from build123d import *

# Parameters (mm, degrees)
SKETCH1_W                = 4.5
SKETCH1_H                = 3.5
BOSS_EXTRUDE1_DEPTH      = 4.5
SKETCH2_W                = 4
SKETCH2_H                = 3
CUT_EXTRUDE1_DEPTH       = 4.25
SKETCH3_R                = 0.15
BOSS_EXTRUDE2_DEPTH      = 2.7
BOSS_EXTRUDE2_DEPTH_BACK = 4
SKETCH4_W                = 3.5
SKETCH4_H                = 0.4
CUT_EXTRUDE2_DEPTH       = 5.5


with BuildPart() as part:
    # Sketch1 → Boss-Extrude1 (new body)
    with BuildSketch(Plane.XY):
        Rectangle(SKETCH1_W, SKETCH1_H)
    extrude(amount=BOSS_EXTRUDE1_DEPTH)

    # Sketch2 → Cut-Extrude1 (cut)
    with BuildSketch(Plane.XY.offset(4.5)):
        Rectangle(SKETCH2_W, SKETCH2_H)
    extrude(amount=-CUT_EXTRUDE1_DEPTH, mode=Mode.SUBTRACT)

    # Sketch3 → Boss-Extrude2 (add, two sides)
    with BuildSketch(Plane(origin=(0, 0, 0), x_dir=(-1, 0, 0), z_dir=(0, 0, -1))) as boss_extrude2_sk:
        with Locations((-0.75, -0.45)):
            Circle(SKETCH3_R)
        with Locations((0.75, -0.45)):
            Circle(SKETCH3_R)
    extrude(amount=BOSS_EXTRUDE2_DEPTH)
    extrude(boss_extrude2_sk.sketch, amount=-BOSS_EXTRUDE2_DEPTH_BACK)

    # Sketch4 → Cut-Extrude2 (cut, through all)
    with BuildSketch(Plane.ZY.offset(2.25)):
        with Locations((4.5, -0.45)):
            Rectangle(SKETCH4_W, SKETCH4_H)
    extrude(amount=-CUT_EXTRUDE2_DEPTH, mode=Mode.SUBTRACT)


solid = part.part
CAD build for the part. Positions are in the model's coordinates, mm. A direction names the side the tool comes from. Coordinates: 2 decimals unless noted, no trailing zeros. Order: outer loops, then holes, each group sorted by start corner. A loop starts at its lowest first (then second) coordinate and runs counter-clockwise, first axis right, second up.
Item 1: Two-plate mould, pull along X, no slides. Class faces 1 (the face through (0, 1.75, 2)), 2 (the face through (0, 1.5, 2)), 3 (the face through (-2, 0, 2)), 4 (the face through (2.25, 0, 2)): +X half, -X half, draft (parallel to the pull), parting line (faces both ways), or undercut.
Check sheet entries:
face 1: draft
face 2: undercut
face 3: undercut
face 4: +X half
Item 2: Drill centre lines: L1, parallel to X at y = 0.95, z = 2.75; L2, parallel to Y at x = -1.85, z = 2.5; L3, parallel to Z at x = 0.25, y = -1.1. Where is each one in solid material? Low to high.
Check sheet entries:
L1: x = -2.25 to -2, 2 to 2.25
L2: y = -1.75 to -1.5, 1.5 to 1.75
L3: z = 0 to 0.25
Item 3: Band-saw the part on C-C on y = -1.15. List the corners of the cut face in (x, z).
Check sheet entries:
outline: (-2.25, 0) - (2.25, 0) - (2.25, 4.5) - (2, 4.5) - (2, 0.25) - (-2, 0.25) - (-2, 4.5) - (-2.25, 4.5) - close
Item 4: Band-saw the part on D-D on x = 0.4. List the corners of the cut face in (y, z).
Check sheet entries:
outline: (-1.75, 0) - (1.75, 0) - (1.75, 4.5) - (1.5, 4.5) - (1.5, 0.25) - (-1.5, 0.25) - (-1.5, 4.5) - (-1.75, 4.5) - close
Item 5: Band-saw the part on A-A on z = 2.5. List the corners of the cut face in (x, y), plus the area to 3 significant figures.
Check sheet entries:
outline: (-2.25, -1.75) - (2.25, -1.75) - (2.25, 1.75) - (-2.25, 1.75) - close; circle Ø0.3 at (-0.75, -0.45); circle Ø0.3 at (0.75, -0.45); hole (-2, -1.5) - (2, -1.5) - (2, 1.5) - (-2, 1.5) - close
area: 3.89 mm2
Item 6: Band-saw the part on B-B on z = 4.25. List the corners of the cut face in (x, y).
Check sheet entries:
outline: (-2.25, -1.75) - (2.25, -1.75) - (2.25, -0.65) - (2, -0.65) - (2, -1.5) - (-2, -1.5) - (-2, -0.65) - (-2.25, -0.65) - close; (-2.25, -0.25) - (-2, -0.25) - (-2, 1.5) - (2, 1.5) - (2, -0.25) - (2.25, -0.25) - (2.25, 1.75) - (-2.25, 1.75) - close
Item 7: 3-axis set-ups, long thin cutter, end or side, ignore diameter. For faces 5 (the face through (0, -1.75, 2)), 6 (the face through (0, 0, 0.25)): which of +Z, -Z, +X, -X, +Y, -Y reach the whole face in a straight line?
Check sheet entries:
face 5: +Z, -Z, +X, -X, -Y
face 6: +Z
Item 8: Pin check, flat tips, straight feed: pin 1 Ø0.9 at (y, z) = (-0.5, 3) entering from +X; pin 2 Ø0.9 at (x, y) = (-0.5, 0) entering from +Z; pin 3 Ø1 at (x, y) = (0, 0.5) entering from -Z. Stop position of each tip, or through.
Check sheet entries:
pin 1: stops at x = 2.25
pin 2: stops at z = 2.75
pin 3: stops at z = 0
